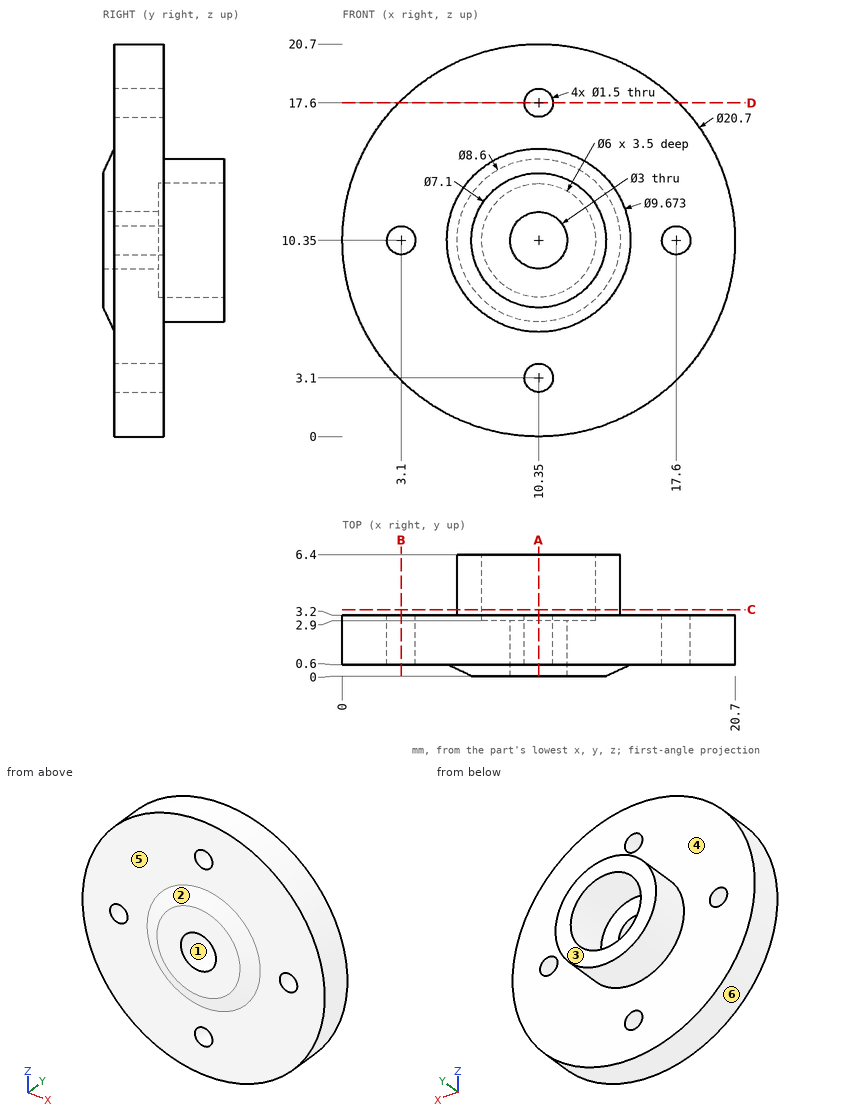
Here's the drawing with two shaded views (mm, measured from the low corner). I have some questions. A direction names the side the tool comes from. Give positions to 0.01 mm unless a question says otherwise; leave off trailing zeros. Loops run counter-clockwise (first coordinate to the right, second up) from the corner with the lowest first, then second, coordinate; pieces in that order, holes last. Notation, with made-up numbers: (-7, -21) -> (39, -21) arc R12 cw to (39, 2) -> close; hole circle Ø6 at (-37, 85.25). An arc over 180 degrees is marked (long way). Answer as a JSON object with one key per item and string values. Group by question number.
Item 1: On a 3-axis mill with a long thin cutter (end or side, diameter ignored), from which of +Z, -Z, +X, -X, +Y, -Y can I reach the whole of each face in a straight line? I mean the marked faces 4, 5 and 6. Say none if no direction works.
Item 2: Imagine slicing it at D-D on z = 17.6. Write out the boundary of the cut face in (x, y), then the cut area to 3 significant figures.
Item 3: Imagine slicing it at B-B on x = 3.1. Write out the boundary of the cut face in (y, z), then the cut area to 3 significant figures.
Item 4: Will these pins go through, and if not, where does the flat tip stop? pin 1 (6 mm diameter, centred on x = 18, z = 2.5, fed in from -Y); pin 2 (1.4 mm diameter, centred on x = 17.6, z = 10.35, fed in from +Y); pin 3 (4 mm diameter, centred on x = 10.35, z = 10.35, fed in from +Y); pin 4 (2 mm diameter, centred on y = 1, z = 7.5, fed in from +X).
Item 5: Imagine slicing it at C-C on y = 3.5. Write out the boundary of the cut face in (x, z).
Item 6: Thinking about a two-plate mould opening in X: for the marked faces 1, 2 and 3, which applies, pulls with the +X half, pulls with the -X half, needs draft (parallel to the pull), parting line crosses it, or undercut?
Item 7: I need wall thicknesses on L1, parallel to X at y = 1.5, z = 10.35; L2, parallel to Z at x = 10.5, y = 2 (1 decimal); L3, parallel to Y at x = 12.25, z = 15.5. Which ranges of each line are inside material? Lowest first, please.
Item 8: Imagine slicing it at A-A on x = 10.35. Write out the boundary of the cut face in (y, z).
Answer list:
{
 "1": {"face 4": "+Y", "face 5": "-Y", "face 6": "+Y, -Y"},
 "2": {"outline": "(2.96, 0.6) -> (9.6, 0.6) -> (9.6, 3.2) -> (2.96, 3.2) -> close; (11.1, 0.6) -> (17.74, 0.6) -> (17.74, 3.2) -> (11.1, 3.2) -> close", "area": "34.5 mm2"},
 "3": {"outline": "(0.6, 2.96) -> (3.2, 2.96) -> (3.2, 9.6) -> (0.6, 9.6) -> close; (0.6, 11.1) -> (3.2, 11.1) -> (3.2, 17.74) -> (0.6, 17.74) -> close", "area": "34.5 mm2"},
 "4": {"pin 1": "stops at y = 0.6", "pin 2": "passes through", "pin 3": "stops at y = 2.9", "pin 4": "stops at x = 20.53"},
 "5": {"outline": "circle Ø8.6 at (10.35, 10.35); hole circle Ø6 at (10.35, 10.35)"},
 "6": {"face 1": "undercut", "face 2": "parting line crosses it", "face 3": "needs draft"},
 "7": {"L1": "x = 0 to 2.35, 3.85 to 8.85, 11.85 to 16.85, 18.35 to 20.7", "L2": "z = 0 to 2.4, 3.8 to 8.9, 11.8 to 16.9, 18.3 to 20.7", "L3": "y = 0.6 to 3.2"},
 "8": {"outline": "(0, 6.8) -> (0.6, 5.51) -> (0.6, 3.85) -> (3.2, 3.85) -> (3.2, 6.05) -> (6.4, 6.05) -> (6.4, 7.35) -> (2.9, 7.35) -> (2.9, 8.85) -> (0, 8.85) -> close; (0, 11.85) -> (2.9, 11.85) -> (2.9, 13.35) -> (6.4, 13.35) -> (6.4, 14.65) -> (3.2, 14.65) -> (3.2, 16.85) -> (0.6, 16.85) -> (0.6, 15.19) -> (0, 13.9) -> close; (0.6, 0) -> (3.2, 0) -> (3.2, 2.35) -> (0.6, 2.35) -> close; (0.6, 18.35) -> (3.2, 18.35) -> (3.2, 20.7) -> (0.6, 20.7) -> close"}
}
